```python
from build123d import *

# Parameters (mm, degrees)
CROQUIS1_W              = 100
CROQUIS1_H              = 100
SALIENTE_EXTRUIR1_DEPTH = 30
CROQUIS2_R              = 1.5
CORTAR_EXTRUIR1_DEPTH   = 38
CROQUIS3_W              = 7.071067812
CROQUIS3_H              = 7.071067812
CORTAR_EXTRUIR2_DEPTH   = 28
VACIADO1_START          = -48
VACIADO1_OUTLINE_W      = 28
VACIADO1_OUTLINE_H      = 81.857864376
VACIADO1_DEPTH          = 96
VACIADO1_START_2        = -40.928932188
VACIADO1_2_OUTLINE_W    = 28
VACIADO1_2_OUTLINE_H    = 7.071067812
VACIADO1_2_DEPTH        = 81.857864376


# Read off the part's stored shape, not the designer's step: Vaciado1
with BuildPart() as part:
    # Croquis1 → Saliente-Extruir1 (new body)
    with BuildSketch(Plane(origin=(0, 0, 0), x_dir=(1, 0, 0), z_dir=(0, 1, 0))):
        Rectangle(CROQUIS1_W, CROQUIS1_H)
    extrude(amount=SALIENTE_EXTRUIR1_DEPTH)

    # Croquis2 → Cortar-Extruir1 (cut)
    with BuildSketch(Plane(origin=(0, 30, 0), x_dir=(1, 0, 0), z_dir=(0, 1, 0))):
        with Locations(Location((-46.464466094, -46.464466094, 0), (0, 0, 270))):
            Circle(CROQUIS2_R)
        with Locations(Location((-46.464466094, 46.464466094, 0), (0, 0, 270))):
            Circle(CROQUIS2_R)
        with Locations(Location((46.464466094, 46.464466094, 0), (0, 0, 270))):
            Circle(CROQUIS2_R)
        with Locations(Location((46.464466094, -46.464466094, 0), (0, 0, 270))):
            Circle(CROQUIS2_R)
    extrude(amount=-CORTAR_EXTRUIR1_DEPTH, mode=Mode.SUBTRACT)

    # Croquis3 → Cortar-Extruir2 (cut)
    with BuildSketch(Plane(origin=(0, 30, 0), x_dir=(1, 0, 0), z_dir=(0, 1, 0))):
        with Locations((-46.464466094, -46.464466094)):
            Rectangle(CROQUIS3_W, CROQUIS3_H)
        with Locations((-46.464466094, 46.464466094)):
            Rectangle(CROQUIS3_W, CROQUIS3_H)
        with Locations((46.464466094, 46.464466094)):
            Rectangle(CROQUIS3_W, CROQUIS3_H)
        with Locations((46.464466094, -46.464466094)):
            Rectangle(CROQUIS3_W, CROQUIS3_H)
    extrude(amount=-CORTAR_EXTRUIR2_DEPTH, mode=Mode.SUBTRACT)

    # Vaciado1 outline → Vaciado1 (cut)
    with BuildSketch(Plane.YZ.offset(VACIADO1_START)):
        with Locations((14, 0)):
            Rectangle(VACIADO1_OUTLINE_W, VACIADO1_OUTLINE_H)
    extrude(amount=VACIADO1_DEPTH, mode=Mode.SUBTRACT)

    # Vaciado1 2 outline → Vaciado1 2 (cut)
    with BuildSketch(Plane.YZ.offset(VACIADO1_START_2)):
        with Locations((14, -44.464466094)):
            Rectangle(VACIADO1_2_OUTLINE_W, VACIADO1_2_OUTLINE_H)
        with Locations((14, 44.464466094)):
            Rectangle(VACIADO1_2_OUTLINE_W, VACIADO1_2_OUTLINE_H)
    extrude(amount=VACIADO1_2_DEPTH, mode=Mode.SUBTRACT)


solid = part.part
```
Design review of the part built by this model. Coordinates are the model's own, in mm. A direction names the side the tool comes from. Give positions to 0.01 mm unless a question says otherwise; leave off trailing zeros. Write each loop counter-clockwise with the first axis right and the second up, starting at its lowest first coordinate (ties: lowest second). Pieces come first, ordered by that corner, then holes.
(1) Add section C-C (x = -33). Give the boundary of the cut face in (y, z), and give its area (3 significant figures).
Checked values:
outline: (0, -50) - (30, -50) - (30, 50) - (0, 50) - (0, 48) - (28, 48) - (28, -48) - (0, -48) - close
area: 312 mm2
(2) Wall thickness on line 1 along X through (y, z) = (21.25, -15.5); line 2 along X through (y, z) = (5.25, 44): over which ranges is each line inside the solid? List them lowest first.
Checked values:
line 1: x = -50 to -48, 48 to 50
line 2: x = -42.93 to -40.93, 40.93 to 42.93
(3) Add section A-A (y = 9.75). Give the boundary of the cut face in (x, z).
Checked values:
outline: (-50, -42.93) - (-42.93, -42.93) - (-42.93, -50) - (42.93, -50) - (42.93, -42.93) - (50, -42.93) - (50, 42.93) - (42.93, 42.93) - (42.93, 50) - (-42.93, 50) - (-42.93, 42.93) - (-50, 42.93) - close; hole (-48, -40.93) - (-40.93, -40.93) - (-40.93, -48) - (40.93, -48) - (40.93, -40.93) - (48, -40.93) - (48, 40.93) - (40.93, 40.93) - (40.93, 48) - (-40.93, 48) - (-40.93, 40.93) - (-48, 40.93) - close
(4) Clearance check with flat-ended pins moving along their axes: pin 1 Ø8 at (y, z) = (18.5, 48) entering from +X; pin 2 Ø1 at (x, z) = (21, 37.5) entering from -Y; pin 3 Ø5.5 at (x, y) = (47.5, 17.5) entering from -Z. State where each tip first meets the part, or that it passes through.
Checked values:
pin 1: stops at x = 42.93
pin 2: stops at y = 28
pin 3: stops at z = -42.93
(5) Tool access review of faces 1 (the face through (40.929, 14, 45)), 2 (the face through (44.8, 2, -46.5)), 3 (the face through (-42.929, 16, -46)), 4 (the face through (-42.929, 16, 47)): name each direction out of +Z, -Z, +X, -X, +Y, -Y from which nothing blocks a thin tool from reaching the whole face with its end or side.
Checked values:
face 1: -Y
face 2: -Z, +X, +Y
face 3: -Z, -X, +Y
face 4: +Z, -X, +Y
(6) Mouldability with a two-part tool opening along X and no side actions: class faces 5 (the face through (44, 14, 40.929)), 6 (the face through (-45, 14, -40.929)), 7 (the face through (42.929, 16, -46)), 8 (the face through (-1, 15, -50)) as +X half, -X half, draft (parallel to the pull), parting line (faces both ways), or undercut.
Checked values:
face 5: undercut
face 6: undercut
face 7: +X half
face 8: draft
(7) Add section B-B (z = -16). Give the boundary of the cut face in (x, y).
Checked values:
outline: (-50, 0) - (-48, 0) - (-48, 28) - (48, 28) - (48, 0) - (50, 0) - (50, 30) - (-50, 30) - close
